Can you work these out from the model? Positions are in its coordinate system, mm. A direction names the side the tool comes from. Round coordinates to 2 decimals unless told otherwise and drop trailing zeros. Loops run counter-clockwise (first coordinate to the right, second up) from the corner with the lowest first, then second, coordinate; pieces in that order, holes last. Notation, with made-up numbers: (-8, -20) -> (14, -20) arc R17 ccw to (14, -13) -> close; hole circle Ø2 at (-37, -6.75). An arc over 180 degrees is marked (long way). Write item = value, one per line.
from build123d import *

# Parameters (mm, degrees)
SKETCH1_W           = 7.62
SKETCH1_H           = 16.47698
BOSS_EXTRUDE1_DEPTH = 3.175
SKETCH2_W           = 3.175
SKETCH2_H           = 1.8796
CUT_EXTRUDE1_DEPTH  = 3.175


with BuildPart() as part:
    # Sketch1 → Boss-Extrude1 (new body)
    with BuildSketch(Plane.XY):
        with Locations((3.81, 8.23849)):
            Rectangle(SKETCH1_W, SKETCH1_H)
    extrude(amount=BOSS_EXTRUDE1_DEPTH)

    # Sketch2 → Cut-Extrude1 (cut)
    with BuildSketch(Plane.XY.offset(3.175)):
        Polygon((2.8702, 11.05789), (4.7498, 11.05789), (4.7498, 9.17829), (6.6294, 9.17829), (6.6294, 7.29869), (4.7498, 7.29869), (4.7498, 5.41909), (2.8702, 5.41909), (2.8702, 7.29869), (0.9906, 7.29869), (0.9906, 9.17829), (2.8702, 9.17829), align=None)
        with Locations((3.81, 15.090268823)):
            Rectangle(SKETCH2_W, SKETCH2_H)
        with Locations((3.81, 1.386968823)):
            Rectangle(SKETCH2_W, SKETCH2_H)
    extrude(amount=-CUT_EXTRUDE1_DEPTH, mode=Mode.SUBTRACT)


solid = part.part
1. For faces 4 (the flat face through (5, 10, 0)), 5 (the flat face through (5.398, 1, 2)), which set-ups out of +Z, -Z, +X, -X, +Y, -Y let a thin tool reach every point of the face, with its end or its side?
Entries:
face_4 = -Z, +X, -X, +Y, -Y
face_5 = +Z, -Z
2. We'd pull the mould along Y, two halves only. Please class faces 1 (the flat face through (2.222, 15, 2)), 2 (the flat face through (4, 0, 2)), 3 (the flat face through (5, 10, 3.175)): released by +Y, released by -Y, zero draft, split by the parting line, or undercut.
Entries:
face_1 = undercut
face_2 = released by -Y
face_3 = zero draft
3. Suppose I cut it at D-D, the plane z = 1.8. List the corners of the cut face in (x, y) for me.
Entries:
outline = (0, 0) -> (7.62, 0) -> (7.62, 16.48) -> (0, 16.48) -> close; hole (0.99, 7.3) -> (2.87, 7.3) -> (2.87, 5.42) -> (4.75, 5.42) -> (4.75, 7.3) -> (6.63, 7.3) -> (6.63, 9.18) -> (4.75, 9.18) -> (4.75, 11.06) -> (2.87, 11.06) -> (2.87, 9.18) -> (0.99, 9.18) -> close; hole (2.22, 0.45) -> (5.4, 0.45) -> (5.4, 2.33) -> (2.22, 2.33) -> close; hole (2.22, 14.15) -> (5.4, 14.15) -> (5.4, 16.03) -> (2.22, 16.03) -> close
4. Suppose I cut it at A-A, the plane y = 9.75. List the corners of the cut face in (x, z) for me (3 decimals).
Entries:
outline = (0, 0) -> (2.87, 0) -> (2.87, 3.175) -> (0, 3.175) -> close; (4.75, 0) -> (7.62, 0) -> (7.62, 3.175) -> (4.75, 3.175) -> close
5. Suppose I cut it at C-C, the plane x = 6.25. List the corners of the cut face in (y, z) for me (3 decimals), and give its area (3 significant figures).
Entries:
outline = (0, 0) -> (7.299, 0) -> (7.299, 3.175) -> (0, 3.175) -> close; (9.178, 0) -> (16.477, 0) -> (16.477, 3.175) -> (9.178, 3.175) -> close
area = 46.3 mm²
6. I need wall thicknesses on line 1 (Y direction, x = 2.5, z = 2.35); line 2 (X direction, y = 8.25, z = 2.05); line 3 (Y direction, x = 3, z = 3). Which ranges of each line are inside material? Lowest first, please. Write a range as [from, to].
Entries:
line_1 = [0, 0.45], [2.33, 7.3], [9.18, 14.15], [16.03, 16.48]
line_2 = [0, 0.99], [6.63, 7.62]
line_3 = [0, 0.45], [2.33, 5.42], [11.06, 14.15], [16.03, 16.48]
7. Suppose I cut it at B-B, the plane x = 4.5. List the corners of the cut face in (y, z) for me (3 decimals), and give its area (3 significant figures).
Entries:
outline = (0, 0) -> (0.447, 0) -> (0.447, 3.175) -> (0, 3.175) -> close; (2.327, 0) -> (5.419, 0) -> (5.419, 3.175) -> (2.327, 3.175) -> close; (11.058, 0) -> (14.15, 0) -> (14.15, 3.175) -> (11.058, 3.175) -> close; (16.03, 0) -> (16.477, 0) -> (16.477, 3.175) -> (16.03, 3.175) -> close
area = 22.5 mm²
